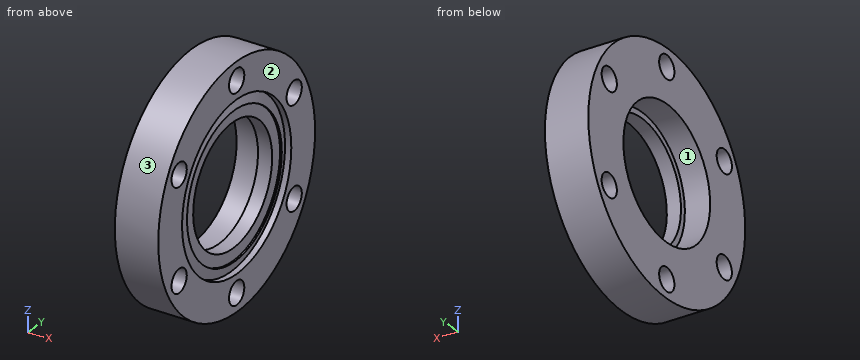
```python
from build123d import *

# Parameters (mm, degrees)
F_1_4_CLEARANCE_HOLE1_D     = 6.731
F_1_4_CLEARANCE_HOLE1_DEPTH = 12.7


with BuildPart() as part:
    # Sketch1 → Revolve1 (revolve)
    with BuildSketch(Plane(origin=(0, 0, 0), x_dir=(-1, 0, 0), z_dir=(0, 0, -1))):
        Polygon((-5.18, 20.95), (-5.18, 0), (6.35, 0), (6.35, 34.671), (-6.35, 34.671), (-6.35, 24.15), (-4.525295248, 24.15), (-5.690000002, 20.95), align=None)
    revolve(axis=Axis((6.35, 0, 0), (-1, 0, 0)))

    # Sketch2 → 1-3/8-6 Tapped Hole1 (revolve, cut)
    with BuildSketch(Plane(origin=(5.18, 0, 0), x_dir=(0, 0, -1), z_dir=(0, 1, 0))):
        Polygon((0, 0), (0, 11.53), (19.177, 11.53), (19.177, 4.1386), (17.4625, 4.1386), (17.4625, 0), align=None)
    revolve(axis=Axis((11.53, 0, 0), (-1, 0, 0)), mode=Mode.SUBTRACT)

    # 1/4 Clearance Hole1
    with Locations(Plane.ZY.offset(6.35)):
        with Locations((14.6812, -25.428584316), (29.3624, 0), (14.6812, 25.428584316), (-14.6812, 25.428584316), (-14.6812, -25.428584316), (-29.3624, 0)):
            Hole(F_1_4_CLEARANCE_HOLE1_D / 2, depth=F_1_4_CLEARANCE_HOLE1_DEPTH)


solid = part.part
```
Input: part model. Units: mm. Frame: model coordinates. Face numbers are marked on the shaded views. Round coordinates to 2 decimals unless told otherwise and drop trailing zeros. Loops run counter-clockwise (first coordinate to the right, second up) from the corner with the lowest first, then second, coordinate; pieces in that order, holes last. Notation, with made-up numbers: M 10,63 L 61,63 A28 ccw 61,92 Z; hole C -33,77.5 d1. An arc over 180 degrees is marked long. Answer in a Markdown table with one row per item. Add a question column.
1. Contact query for flat-ended pins moving along their axis: pin 1 (1 mm diameter, centred on x = -3.5, y = 16.5, fed in from +Z); pin 2 (11.5 mm diameter, centred on y = -8, z = 5.5, fed in from -X); pin 3 (6 mm diameter, centred on y = 16, z = 10, fed in from +X); pin 4 (5 mm diameter, centred on x = 1.5, y = -5, fed in from -Z). Output: stop coordinate, or through.
2. Ray query, probe 1 along Z at (x, y) = (-3, 24); probe 2 along Z at (x, y) = (-4.5, 0.5); probe 3 along Y at (x, z) = (-5, 12.5). Return the intervals inside material, ascending.
3. Section B-B (z = 0). Output: boundary loops of the cut face in (x, y).
4. Section D-D (y = 28). Output: boundary loops of the cut face in (x, z), and give its area (3 significant figures).
5. Section C-C (x = -2). Output: boundary loops of the cut face in (y, z).
6. Section A-A (y = 0). Output: boundary loops of the cut face in (x, z), and give its area (3 significant figures).
7. Mould query, pull axis Z, two halves, no side actions, for the marked faces 1, 2 and 3. Classes: released by +Z, released by -Z, zero draft, split by the parting line, or undercut.
Values follow:
| question | item | result |
|---|---|---|
| 1 | pin 1 | z = 30.76 |
| 1 | pin 2 | through |
| 1 | pin 3 | x = 5.69 |
| 1 | pin 4 | z = -34.58 |
| 2 | probe 1 | -25.02 to -17.73, -11.63 to 11.63, 17.73 to 25.02 |
| 2 | probe 2 | -34.67 to -32.69, -26.03 to -19.17, 19.17 to 26.03, 32.69 to 34.67 |
| 2 | probe 3 | -32.34 to -27.99, -22.87 to -14.54, 14.54 to 22.87, 27.99 to 32.34 |
| 3 | outline | M -6.35,-34.67 L 6.35,-34.67 L 6.35,-24.15 L 4.53,-24.15 L 5.69,-20.95 L 5.18,-20.95 L 5.18,-17.46 L 1.04,-17.46 L 1.04,-19.18 L -6.35,-19.18 Z; M -6.35,19.18 L 1.04,19.18 L 1.04,17.46 L 5.18,17.46 L 5.18,20.95 L 5.69,20.95 L 4.53,24.15 L 6.35,24.15 L 6.35,34.67 L -6.35,34.67 Z |
| 4 | outline | M -6.35,-20.45 L 6.35,-20.45 L 6.35,-16.85 L -6.35,-16.85 Z; M -6.35,-12.51 L 6.35,-12.51 L 6.35,12.51 L -6.35,12.51 Z; M -6.35,16.85 L 6.35,16.85 L 6.35,20.45 L -6.35,20.45 Z |
| 4 | area | 409 mm^2 |
| 5 | outline | C 0,0 d69.34; hole C -25.43,-14.68 d6.73; hole C -25.43,14.68 d6.73; hole C 0,0 d38.35; hole C 0,-29.36 d6.73; hole C 0,29.36 d6.73; hole C 25.43,-14.68 d6.73; hole C 25.43,14.68 d6.73 |
| 6 | outline | M -6.35,-34.67 L 6.35,-34.67 L 6.35,-32.73 L -6.35,-32.73 Z; M -6.35,-26 L 6.35,-26 L 6.35,-24.15 L 4.53,-24.15 L 5.69,-20.95 L 5.18,-20.95 L 5.18,-17.46 L 1.04,-17.46 L 1.04,-19.18 L -6.35,-19.18 Z; M -6.35,19.18 L 1.04,19.18 L 1.04,17.46 L 5.18,17.46 L 5.18,20.95 L 5.69,20.95 L 4.53,24.15 L 6.35,24.15 L 6.35,26 L -6.35,26 Z; M -6.35,32.73 L 6.35,32.73 L 6.35,34.67 L -6.35,34.67 Z |
| 6 | area | 225 mm^2 |
| 7 | face 1 | undercut |
| 7 | face 2 | zero draft |
| 7 | face 3 | split by the parting line |
